from build123d import *

# Parameters (mm, degrees)
F1_DEPTH    = 12.7
F3_DEPTH    = 88.9
F4_T1_DEPTH = 50.8
F5_R        = 5.08


# Not quite as in the source:
# - a fillet or chamfer that OpenCascade refuses, or shapes differently, is made with other operations: its cross-section is extruded or revolved along the edge and cut away or added
# - a feature names something its author has since deleted; it is built from what else it names


with BuildPart() as f1:
    # F0 (on Top) → F1 (new body)
    with BuildSketch(Plane.XY):
        Polygon((10.16, 12.7), (10.16, -12.7), (-10.16, -12.7), (-10.16, 12.7), (-10.16, 22.225), (-19.685, 22.225), (-19.685, -22.225), (19.685, -22.225), (19.685, 22.225), (10.16, 22.225), align=None)
    extrude(amount=-F1_DEPTH)

    # F2 (on face) → F3 (join)
    with BuildSketch(Plane.XY):
        Polygon((-12.7, -12.7), (-12.7, -22.225), (12.7, -22.225), (12.7, -12.7), (10.16, -12.7), (-10.16, -12.7), align=None)
    extrude(amount=F3_DEPTH)

    # F4: fillet of radius 5.08 on 2 edges, made by hand

    # F4_s2 → F4_t1 (cut)
    with BuildSketch(Plane.YZ.offset(-25.4)):
        with BuildLine():
            ThreePointArc((-12.7, 83.82), (-14.1878975516, 87.4121024484), (-17.78, 88.9))
            Line((-17.78, 88.9), (-12.7, 88.9))
            Line((-12.7, 88.9), (-12.7, 83.82))
        make_face()
        with BuildLine():
            ThreePointArc((-22.225, 83.82), (-20.7371024484, 87.4121024484), (-17.145, 88.9))
            Line((-17.145, 88.9), (-22.225, 88.9))
            Line((-22.225, 88.9), (-22.225, 83.82))
        make_face()
    extrude(amount=F4_T1_DEPTH, mode=Mode.SUBTRACT)

    # F5
    f5_edges = [f1.edges().sort_by_distance(p)[0] for p in [
        (14.9225, 22.225, -12.7),
        (-14.9225, 22.225, -12.7),
    ]]
    fillet(f5_edges, radius=F5_R)


solid = f1.part
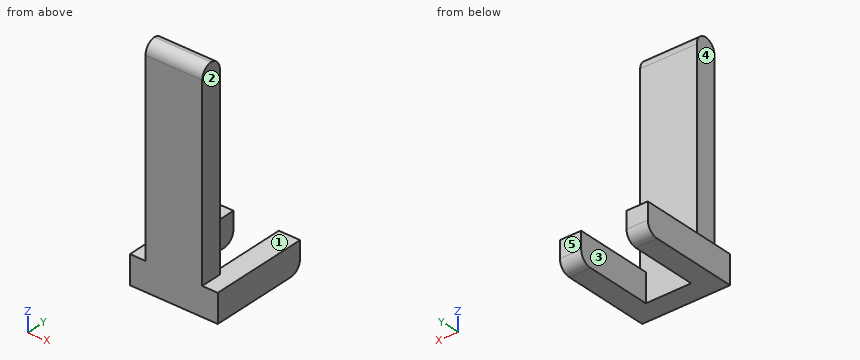
The listing builds one solid part. Answer for the finished solid, in the listing's coordinates (mm). Face numbers are marked on the shaded views. A direction names the side the tool comes from. Give positions to 0.01 mm unless a question says otherwise; leave off trailing zeros. Loops run counter-clockwise (first coordinate to the right, second up) from the corner with the lowest first, then second, coordinate; pieces in that order, holes last. Notation, with made-up numbers: (6, 50.25) - (36, 50.25) arc R18 ccw to (36, 77.25) - close; hole circle Ø10 at (69, 46.25). An arc over 180 degrees is marked (long way). Write each question's results on one line, items separated by ' | '.
1. Flat-ended cylindrical pins translate along their axes: P1, Ø3, axis at x = -14, y = 6.5, coming from the +Z side; P2, Ø1, axis at x = 1, z = 34, coming from the +Y side; P3, Ø10.5, axis at y = -15.5, z = 61, coming from the +X side; P4, Ø10, axis at x = -2.5, y = 11, coming from the +Z side. Find the tip coordinate at first contact, or state that the pin passes through.
Resolved:
P1: stops at z = 0 | P2: stops at y = -12.7 | P3: stops at x = 12.7 | P4: passes through
2. Find section A-A, the plane y = 12. Write down the section's boundary in (x, z) (3 decimals), then the cut area to 3 significant figures.
Resolved:
outline: (-19.685, -12.7) - (-10.16, -12.7) - (-10.16, 0) - (-19.685, 0) - close; (10.16, -12.7) - (19.685, -12.7) - (19.685, 0) - (10.16, 0) - close | area: 242 mm^2
3. Find section B-B, the plane z = -5. Write down the section's boundary in (x, y) (3 decimals).
Resolved:
outline: (-19.685, -22.225) - (19.685, -22.225) - (19.685, 22.225) - (10.16, 22.225) - (10.16, -12.7) - (-10.16, -12.7) - (-10.16, 22.225) - (-19.685, 22.225) - close
4. Which of the six approach directions +Z, -Z, +X, -X, +Y, -Y give full straight-line access (tool end or side, diameter ignored) to the marked faces 1, 2, 3, 4 and 5?
Resolved:
face 1: +Z, +X, +Y | face 2: +Z, +X, +Y, -Y | face 3: +Z, -Z, +Y | face 4: +Z, -X, +Y, -Y | face 5: +Z, -Z, +X, -X, +Y
5. Find section D-D, the plane y = 19. Write down the section's boundary in (x, z) (3 decimals), then the cut area to 3 significant figures.
Resolved:
outline: (-19.685, -12.349) - (-10.16, -12.349) - (-10.16, 0) - (-19.685, 0) - close; (10.16, -12.349) - (19.685, -12.349) - (19.685, 0) - (10.16, 0) - close | area: 235 mm^2
6. Find section C-C, the plane x = 14. Write down the section's boundary in (y, z) (3 decimals), then the cut area to 3 significant figures.
Resolved:
outline: (-22.225, -12.7) - (17.145, -12.7) arc R5.08 ccw to (22.225, -7.62) - (22.225, 0) - (-22.225, 0) - close | area: 559 mm^2
7. Consider probe 1 along X at (y, z) = (-12, -4.5) (3 decimals); probe 2 along Y at (x, z) = (5, 75) (3 decimals); probe 3 along Z at (x, y) = (11, -10.5). Determine where each line is inside the solid, lowest interval first. Write a range as from..to.
Resolved:
probe 1: x = -19.685..-10.16, 10.16..19.685 | probe 2: y = -22.225..-12.7 | probe 3: z = -12.7..0
